Input: part model. Units: mm. Frame: model coordinates. Give positions to 0.01 mm unless a question says otherwise; leave off trailing zeros. Loops run counter-clockwise (first coordinate to the right, second up) from the corner with the lowest first, then second, coordinate; pieces in that order, holes last. Notation, with made-up numbers: (55.25, 18) -> (96.25, 18) arc R24 cw to (96.25, 57) -> close; hole circle Ø6 at (18.25, 27). An arc over 180 degrees is marked (long way). Answer as a JSON object with one key per item and string values. Group by question number.
Autodesk Inventor part; units mm, degrees
ref_plane "YZ Plane" through (0, 0, 0) normal (1, 0, 0) x (0, 1, 0)
ref_plane "XZ Plane" through (0, 0, 0) normal (0, 1, 0) x (-1, 0, 0)
ref_plane "XY Plane" through (0, 0, 0) normal (0, 0, 1) x (1, 0, 0)
sketch "スケッチ1" plane through (0, 0, 0) normal (0, 0, 1) x (1, 0, 0)
  line L0 (0, 0) -> (80, 0)
  line L1 (80, 0) -> (80, 50)
  line L2 (80, 50) -> (0, 50)
  line L3 (0, 50) -> (0, 0)
  dimension "d0" = 80
  dimension "d1" = 50
extrude "押し出し1" add sketch "スケッチ1" along normal blind 3
sketch "スケッチ2" plane through (0, 0, 3) normal (0, 0, 1) x (1, 0, 0)
  circle A0 centre (40, 25) radius 23.5
  line L0 (0, 0) -> (80, 0)
  line L1 (0, 50) -> (0, 0)
  dimension "d4" = 47
  dimension "d5" = 25
  dimension "d6" = 40
extrude "押し出し2" cut sketch "スケッチ2" against normal blind 3
sketch "スケッチ3" plane through (0, 0, 3) normal (0, 0, 1) x (1, 0, 0)
  circle A0 centre (7.5, 45) radius 1.6
  line L0 (0, 50) -> (0, 0)
  line L1 (80, 50) -> (0, 50)
  circle A1 centre (7.5, 5) radius 1.6
  line L2 (0, 0) -> (80, 0)
  circle A2 centre (72.5, 45) radius 1.6
  line L3 (80, 0) -> (80, 50)
  circle A3 centre (72.5, 5) radius 1.6
  dimension "d9" = 3.2
  dimension "d10" = 7.5
  dimension "d11" = 5
  dimension "d12" = 3.2
  dimension "d13" = 5
  dimension "d14" = 3.2
  dimension "d15" = 7.5
  dimension "d16" = 5
  dimension "d17" = 3.2
  dimension "d18" = 5
  dimension "d19" = 7.5
  dimension "d20" = 7.5
hole "穴1" at (7.5, 45, 3) at (7.5, 5, 3) at (72.5, 45, 3) at (72.5, 5, 3) direction (0, 0, -1) diameter 3.2 depth 3
sketch "スケッチ4" plane through (0, 0, 3) normal (0, 0, 1) x (1, 0, 0)
  point P0 (0, 0)
equation "\"BendRadius\" = Thickness"
equation "\"BendReliefWidth\" = Thickness"
equation "\"BendReliefDepth\" = 0.5 * Thickness"
equation "\"CornerReliefSize\" = 4 * Thickness"
equation "\"MinimumRemnant\" = 2 * Thickness"
equation "\"TransitionRadius\" = BendRadius"
equation "\"JacobiRadiusSize\" = BendRadius"
equation "\"GapSize\" = Thickness"
properties part number "nhk31"
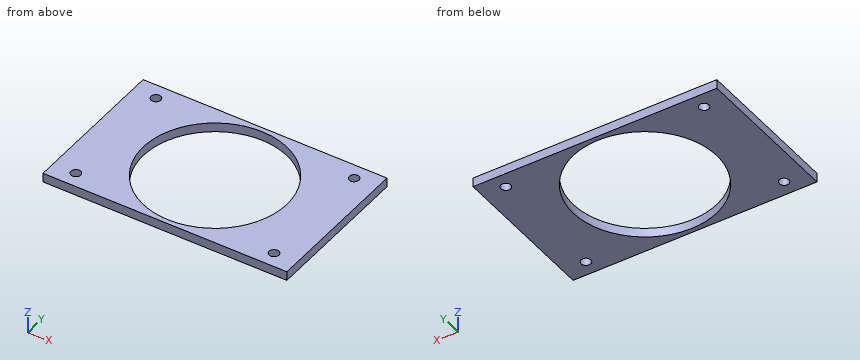
Q1. Section C-C on x = 72.5. Return the cut outline in (y, z).
Q2. Section A-A on y = 25. Return the cut outline in (x, z), then the cut area to 3 significant figures.
Q3. Section D-D on x = 31.5. Return the cut outline in (y, z).
Q4. Section B-B on z = 1.6. Return the cut outline in (x, y).
Q5. Ray query, probe 1 along Y at (x, z) = (72.5, 2); probe 2 along Y at (x, z) = (40, 1.9); probe 3 along X at (y, z) = (45, 2.1). Return the intervals inside material, ascending.
Numbers:
{
 "1": {"outline": "(0, 0) -> (3.4, 0) -> (3.4, 3) -> (0, 3) -> close; (6.6, 0) -> (43.4, 0) -> (43.4, 3) -> (6.6, 3) -> close; (46.6, 0) -> (50, 0) -> (50, 3) -> (46.6, 3) -> close"},
 "2": {"outline": "(0, 0) -> (16.5, 0) -> (16.5, 3) -> (0, 3) -> close; (63.5, 0) -> (80, 0) -> (80, 3) -> (63.5, 3) -> close", "area": "99.0 mm²"},
 "3": {"outline": "(0, 0) -> (3.09, 0) -> (3.09, 3) -> (0, 3) -> close; (46.91, 0) -> (50, 0) -> (50, 3) -> (46.91, 3) -> close"},
 "4": {"outline": "(0, 0) -> (80, 0) -> (80, 50) -> (0, 50) -> close; hole circle Ø3.2 at (7.5, 5); hole circle Ø3.2 at (7.5, 45); hole circle Ø47 at (40, 25); hole circle Ø3.2 at (72.5, 5); hole circle Ø3.2 at (72.5, 45)"},
 "5": {"probe 1": "y = 0 to 3.4, 6.6 to 43.4, 46.6 to 50", "probe 2": "y = 0 to 1.5, 48.5 to 50", "probe 3": "x = 0 to 5.9, 9.1 to 27.66, 52.34 to 70.9, 74.1 to 80"}
}
